from build123d import *

# Parameters (mm, degrees)
F0_R     = 15
F0_R_2   = 10
F1_DEPTH = 25
F2_DEPTH = 50
F3_R     = 2
F4_SIZE  = 3


with BuildPart() as f1:
    # F0 (on Front) → F1 (new body)
    with BuildSketch(Plane.XZ):
        with BuildLine():
            ThreePointArc((6.25, 29.341736), (23.318448, 18.874586), (30, 0))
            ThreePointArc((30, 0), (23.318448, -18.874586), (6.25, -29.341736))
            Line((6.25, -29.341736), (63.645833, -17.116013))
            ThreePointArc((63.645833, -17.116013), (42.5, 0), (63.645833, 17.116013))
            Line((63.645833, 17.116013), (6.25, 29.341736))
        make_face()
        with BuildLine():
            ThreePointArc((6.25, -29.341736), (23.318448, -18.874586), (30, 0))
            ThreePointArc((30, 0), (23.318448, 18.874586), (6.25, 29.341736))
            ThreePointArc((6.25, 29.341736), (-30, 0), (6.25, -29.341736))
        make_face()
        Circle(F0_R, mode=Mode.SUBTRACT)
        with BuildLine():
            ThreePointArc((77.5, 0), (73.602428, 11.010175), (63.645833, 17.116013))
            ThreePointArc((63.645833, 17.116013), (42.5, 0), (63.645833, -17.116013))
            ThreePointArc((63.645833, -17.116013), (73.602428, -11.010175), (77.5, 0))
        make_face()
        with Locations((60, 0)):
            Circle(F0_R_2, mode=Mode.SUBTRACT)
    extrude(amount=F1_DEPTH)

    # F0 (on Front) → F2 (join)
    with BuildSketch(Plane.XZ):
        with BuildLine():
            ThreePointArc((6.25, -29.341736), (23.318448, -18.874586), (30, 0))
            ThreePointArc((30, 0), (23.318448, 18.874586), (6.25, 29.341736))
            ThreePointArc((6.25, 29.341736), (-30, 0), (6.25, -29.341736))
        make_face()
        Circle(F0_R, mode=Mode.SUBTRACT)
    extrude(amount=F2_DEPTH)

    # F3
    f3_edges = [f1.edges().sort_by_distance(p)[0] for p in [
        (34.947917, 0, -23.228875),
        (-6.25, -50, 29.341736),
    ]]
    fillet(f3_edges, radius=F3_R)

    # F4
    f4_edges = [f1.edges().sort_by_distance(p)[0] for p in [
        (50, -25, 0),
        (-15, 0, 0),
        (15, -25, 0),
        (-15, -50, 0),
    ]]
    chamfer(f4_edges, length=F4_SIZE)


solid = f1.part
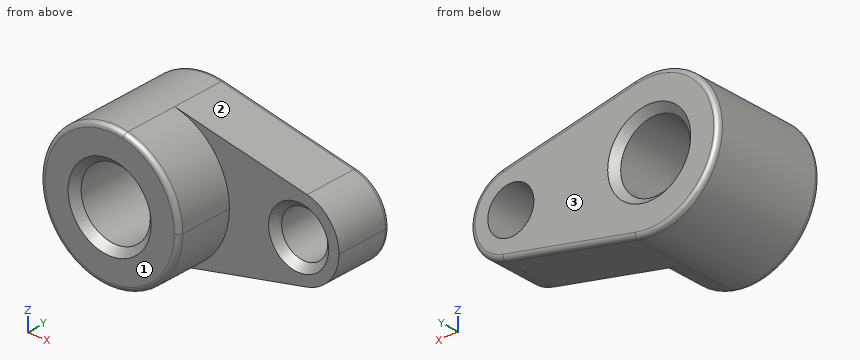
Work out the finished part from the listing and answer in its coordinate system (mm). Face numbers are marked on the shaded views. Give positions to 0.01 mm unless a question says otherwise; leave off trailing zeros. Write each loop counter-clockwise with the first axis right and the second up, starting at its lowest first coordinate (ties: lowest second). Pieces come first, ordered by that corner, then holes. Notation, with made-up numbers: (21, 67.25) - (51, 67.25) arc R22 cw to (51, 80.25) - close; hole circle Ø3 at (-10, 41.5). An arc over 180 degrees is marked (long way). One line per item, written item: value. Start each with the question number.
1. For a pull along Y with two mould halves and no side action, classify the marked faces 1, 2 and 3 as +Y half, -Y half, draft (parallel to the pull), parting line (faces both ways), or undercut.
2. Given pin 1 (5 mm diameter, centred on x = 48, y = -9.5, fed in from +Z); pin 2 (1 mm diameter, centred on y = -6.5, z = -0.5, fed in from -X); pin 3 (4 mm diameter, centred on y = -38, z = -10.5, fed in from +X), each flat-ended and moving along its own axis, determine where each tip first touches the part or whether it passes through.
3. Consider probe 1 along X at (y, z) = (-4.5, -2); probe 2 along Z at (x, y) = (0, -36); probe 3 along X at (y, z) = (-16, 4). Determine where each line is inside the solid, lowest interval first.
4. Find section B-B (y = -27). Write down the section's boundary in (x, z), then the cut area to 3 significant figures.
5. Find section A-A (y = -10.5). Write down the section's boundary in (x, z).
Geometry results:
1. face 1: -Y half
1. face 2: draft
1. face 3: +Y half
2. pin 1: z = 20.98
2. pin 2: x = -30
2. pin 3: x = 28.77
3. probe 1: -29.93 to -14.87, 14.87 to 50.2, 69.8 to 77.39
3. probe 2: -30 to -15, 15 to 30
3. probe 3: -29.73 to -14.46, 14.46 to 50.83, 69.17 to 77.04
4. outline: (6.25, -29.34) arc R30 ccw to (30, 0) arc R30 ccw to (6.25, 29.34) arc R30 ccw (long way) to start; hole circle Ø30 at (0, 0)
4. area: 2,120 mm2
5. outline: (6.25, -29.34) - (63.65, -17.12) arc R17.5 ccw to (63.65, 17.12) - (6.25, 29.34) arc R30 ccw (long way) to start; hole circle Ø30 at (0, 0); hole circle Ø20 at (60, 0)
